Verification items for the finished model (mm, model axes). Round coordinates to 2 decimals unless told otherwise and drop trailing zeros. Write each loop counter-clockwise with the first axis right and the second up, starting at its lowest first coordinate (ties: lowest second). Pieces come first, ordered by that corner, then holes. Notation, with made-up numbers: M 19.5,-11 L 25.5,-11 A11 cw 25.5,2 Z; hole C 86,-1 d6. An arc over 180 degrees is marked long. One line per item, written item: value. Start each with the question number.
Item 1: Section check B-B, the plane x = 27.5. Record the cut outline in (y, z), then the cut area to 3 significant figures.
Item 2: Section check A-A, the plane y = 3.7. State how many separate pieces and enclosed holes the cut face has, then the cut area to 3 significant figures.
Item 3: Section check C-C, the plane z = -85. Record the cut outline in (x, y).
Item 4: Thickness scan on probe 1 along Z at (x, y) = (159.5, 0.7); probe 2 along Z at (x, y) = (55.5, 1.25); probe 3 along Z at (x, y) = (184, 0.45). Record the ranges inside material, lowest first. Write a range as from..to.
Item 5: Gauge pin test, flat ends, axial feed: pin 1 (2.5 mm diameter, centred on x = 192.8, z = -89.07, fed in from -Y); pin 2 (2 mm diameter, centred on x = 70, y = 2.5, fed in from -Z); pin 3 (2 mm diameter, centred on x = 108, y = 1, fed in from -Z). Record the tip position at first contact, or that the pin passes through.
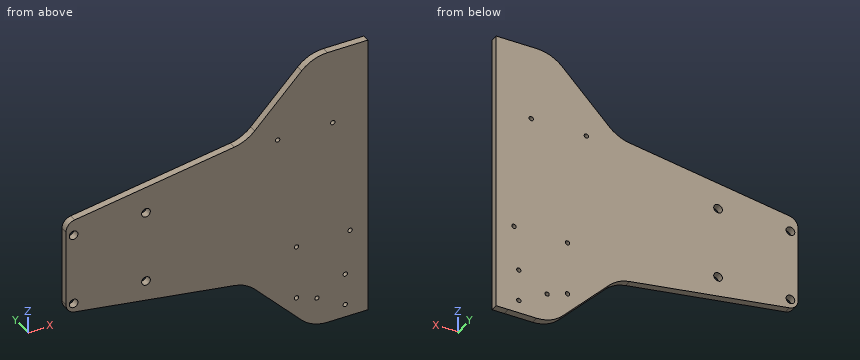
from build123d import *

# Parameters (mm, degrees)
BOSS_EXTRU_1_DEPTH      = 5
CONG_3_R                = 7
ESQUISSE3_R             = 3
ENL_V_MAT_EXTRU_1_DEPTH = 5
ESQUISSE8_R             = 1.5
ENL_V_MAT_EXTRU_5_DEPTH = 10
ESQUISSE11_R            = 1.5
ENL_V_MAT_EXTRU_7_DEPTH = 10
ESQUISSE12_W            = 8.513232075
ESQUISSE12_H            = 196.02308235
BOSS_EXTRU_2_DEPTH      = 5
ESQUISSE13_R            = 1.496707183
ESQUISSE13_R_2          = 1.50175208
ESQUISSE13_R_3          = 1.500339551
ENL_V_MAT_EXTRU_8_DEPTH = 10


with BuildPart() as part:
    # Esquisse1 → Boss.-Extru.1 (new body)
    with BuildSketch(Plane(origin=(0, 0, 0), x_dir=(1, 0, 0), z_dir=(0, 1, 0))):
        with BuildLine():
            Line((200, 98), (180.486918987, 98))
            ThreePointArc((180.486918987, 98), (170.816361757, 96.053857006), (162.651427502, 90.518425828))
            Line((162.651427502, 90.518425828), (130.227508241, 57.507666668))
            ThreePointArc((130.227508241, 57.507666668), (123.786759953, 52.773905469), (116.181163829, 50.314913559))
            Line((116.181163829, 50.314913559), (0, 32.5))
            Line((0, 32.5), (0, 19.62474242))
            Line((0, 19.62474242), (0, -19.62474242))
            Line((0, -19.62474242), (0, -32.5))
            Line((0, -32.5), (116.181163829, -50.314913559))
            ThreePointArc((116.181163829, -50.314913559), (123.786759953, -52.773905469), (130.227508241, -57.507666668))
            Line((130.227508241, -57.507666668), (162.651427502, -90.518425828))
            ThreePointArc((162.651427502, -90.518425828), (170.816361757, -96.053857006), (180.486918987, -98))
            Line((180.486918987, -98), (200, -98))
            Line((200, -98), (200, 98))
        make_face()
    extrude(amount=BOSS_EXTRU_1_DEPTH)

    # Congé3
    cong_3_edges = [part.edges().sort_by_distance(p)[0] for p in [
        (0, 2.5, 32.5),
        (0, 2.5, -32.5),
    ]]
    fillet(cong_3_edges, radius=CONG_3_R)

    # Esquisse3 → Enlèv. mat.-Extru.1 (cut)
    with BuildSketch(Plane(origin=(0, 5, 0), x_dir=(1, 0, 0), z_dir=(0, 1, 0))):
        with Locations((5.228132429, -22.542085275)):
            Circle(ESQUISSE3_R)
        with Locations((5.228132429, 27.05879269)):
            Circle(ESQUISSE3_R)
        with Locations((55.20842969, -22.542085275)):
            Circle(ESQUISSE3_R)
        with Locations((55.20842969, 27.05879269)):
            Circle(ESQUISSE3_R)
    extrude(amount=-ENL_V_MAT_EXTRU_1_DEPTH, mode=Mode.SUBTRACT)

    # Esquisse8 → Enlèv. mat.-Extru.5 (cut)
    with BuildSketch(Plane(origin=(0, 5, 0), x_dir=(1, 0, 0), z_dir=(0, 1, 0))):
        with Locations((196.148923391, 36.274574464)):
            Circle(ESQUISSE8_R)
        with Locations((159.148923391, 73.274574464)):
            Circle(ESQUISSE8_R)
        with Locations((159.148923391, 36.274574464)):
            Circle(ESQUISSE8_R)
    extrude(amount=-ENL_V_MAT_EXTRU_5_DEPTH, mode=Mode.SUBTRACT)

    # Esquisse11 → Enlèv. mat.-Extru.7 (cut)
    with BuildSketch(Plane(origin=(0, 5, 0), x_dir=(1, 0, 0), z_dir=(0, 1, 0))):
        with Locations((184.199116652, -45.869762424)):
            Circle(ESQUISSE11_R)
        with Locations((146.150097665, -45.660518454)):
            Circle(ESQUISSE11_R)
    extrude(amount=-ENL_V_MAT_EXTRU_7_DEPTH, mode=Mode.SUBTRACT)

    # Esquisse12 → Boss.-Extru.2 (add)
    with BuildSketch(Plane(origin=(0, 0, 0), x_dir=(-1, 0, 0), z_dir=(0, -1, 0))):
        with Locations((-204.256616038, 0.011541175)):
            Rectangle(ESQUISSE12_W, ESQUISSE12_H)
    extrude(amount=-BOSS_EXTRU_2_DEPTH)

    # Esquisse13 → Enlèv. mat.-Extru.8 (cut)
    with BuildSketch(Plane(origin=(0, 5, 0), x_dir=(1, 0, 0), z_dir=(0, 1, 0))):
        with Locations((192.801268115, 89.072215784)):
            Circle(ESQUISSE13_R)
        with Locations((173.269117951, 78.05884243)):
            Circle(ESQUISSE13_R_2)
        with Locations((192.801268115, 67.045469076)):
            Circle(ESQUISSE13_R_3)
    extrude(amount=-ENL_V_MAT_EXTRU_8_DEPTH, mode=Mode.SUBTRACT)


solid = part.part
Response values:
1. outline: M 0,-36.72 L 5,-36.72 L 5,36.72 L 0,36.72 Z
1. area: 367 mm2
2. separate pieces: 1
2. enclosed holes: 12
2. area: 24,600 mm2
3. outline: M 157.23,0 L 208.51,0 L 208.51,5 L 157.23,5 Z
4. probe 1: z = -87.31..-74.73, -71.82..-37.73, -34.82..87.31
4. probe 2: z = -41.01..-30.04, -24.07..19.56, 25.53..41.01
4. probe 3: z = -98..44.38, 47.36..98
5. pin 1: passes through
5. pin 2: stops at z = -43.39
5. pin 3: stops at z = -49.21
